from build123d import *

# Parameters (mm, degrees)
F1_W          = 44.750304
F1_H          = 45.399402
F2_R          = 8.174725
F4_DEPTH      = 6.858
F4_DEPTH_BACK = 30.48


with BuildPart() as f3:
    # F1 (on Top) → F3 section 0
    with BuildSketch(Plane.XY, mode=Mode.PRIVATE) as f3_s0:
        Rectangle(F1_W, F1_H)
    loft([f3_s0.sketch, Vertex(0, 0, 40.64)])

    # F2 (on offset) → F4 (join, two sides)
    with BuildSketch(Plane.XY.offset(40.64)) as f4_sk:
        Circle(F2_R)
    extrude(amount=F4_DEPTH)
    extrude(f4_sk.sketch, amount=-F4_DEPTH_BACK)

    # F5 (on face) → F6 (revolve)
    with BuildSketch(Plane.XY.offset(47.498)):
        with BuildLine():
            Line((0, 8.174725), (0, 13.327389))
            ThreePointArc((0, 13.327389), (-13.327389, 0), (0, -13.327389))
            Line((0, -13.327389), (0, -8.174725))
            ThreePointArc((0, -8.174725), (-8.174725, 0), (0, 8.174725))
        make_face()
    revolve(axis=Axis((0, 0, 47.498), (0, -1, 0)))


solid = f3.part
Part model, mm, in its own coordinate system. Coordinates: 2 decimals unless noted, no trailing zeros. Order: outer loops, then holes, each group sorted by start corner. A loop starts at its lowest first (then second) coordinate and runs counter-clockwise, first axis right, second up.
(1) Slice it at A-A, the plane y = 0. Write the cut outline in (x, z).
Check sheet entries:
outline: (-22.38, 0) - (22.38, 0) - (8.17, 25.79) - (8.17, 36.97) arc R13.33 ccw (long way) to (-8.17, 36.97) - (-8.17, 25.79) - close; hole (-8.17, 47.5) - (8.17, 47.5) arc R8.17 ccw to start
(2) Slice it at C-C, the plane y = 11.5. Write the cut outline in (x, z).
Check sheet entries:
outline: (-22.38, 0) - (22.38, 0) - (11.34, 20.05) - (-11.34, 20.05) - close; circle Ø13.47 at (0, 47.5)
(3) Pull direction Y, two halves, no side cores. Call faces 1 (the face through (3.772, -7.252, 31.46)), 2 (the face through (15.79, -0.32, 11.96)), 3 (the face through (-0.31, -16.02, 11.96)), 4 (the face through (0, 0, 47.498)): pulls with the +Y half, pulls with the -Y half, needs draft (parallel to the pull), parting line crosses it, or undercut.
Check sheet entries:
face 1: parting line crosses it
face 2: needs draft
face 3: pulls with the -Y half
face 4: undercut
(4) Slice it at B-B, the plane x = 0. Write the cut outline in (y, z).
Check sheet entries:
outline: (-22.7, 0) - (22.7, 0) - (8.17, 26) - (8.17, 36.97) arc R13.33 ccw (long way) to (-8.17, 36.97) - (-8.17, 26) - close; hole (-8.17, 47.5) - (8.17, 47.5) arc R8.17 ccw to start
(5) Pin check, flat tips, straight feed: pin 1 Ø1.5 at (y, z) = (-15, 11.5) entering from +X; pin 2 Ø6 at (x, z) = (12.5, 21) entering from -Y; pin 3 Ø4 at (x, z) = (12.5, 49) entering from +Y. Stop position of each tip, or through.
Check sheet entries:
pin 1: stops at x = 16.46
pin 2: stops at y = -12.65
pin 3: stops at y = 8.09
(6) Probe L1, parallel to Z at x = 16.5, y = 19.5; L2, parallel to Z at x = -3.5, y = -1; L3, parallel to X at y = 3.5, z = 51.5. List the from-to ranges inside material, lowest first.
Check sheet entries:
L1: z = 0 to 5.73
L2: z = 0 to 47.5, 54.82 to 60.32
L3: x = -12.22 to -6.21, 6.21 to 12.22
(7) Slice it at D-D, the plane x = -19. Write the cut outline in (y, z).
Check sheet entries:
outline: (-22.7, 0) - (22.7, 0) - (19.28, 6.13) - (-19.28, 6.13) - close
